Design review of the part built by this model. Coordinates are the model's own, in mm. A direction names the side the tool comes from. Give positions to 0.01 mm unless a question says otherwise; leave off trailing zeros. Loops run counter-clockwise (first coordinate to the right, second up) from the corner with the lowest first, then second, coordinate; pieces in that order, holes last. Notation, with made-up numbers: (-22, -10) -> (-12, -10) arc R28 cw to (-12, 12) -> close; hole circle Ø10 at (3.5, -31). An arc over 180 degrees is marked (long way). Answer in a Markdown table with one row per item. Add a question column.
(1) For line 1 (X direction, y = -7.5, z = 62.5); line 2 (Y direction, x = -4, z = 11); line 3 (X direction, y = -1.5, z = 25.5), list the stretches that pass through material, from the lowest coordinate up.
(2) For pin 1 (6 mm diameter, centred on y = -4.5, z = 82, fed in from +X); pin 2 (5 mm diameter, centred on x = 5.16, z = 92.08, fed in from -Y); pin 3 (4 mm diameter, centred on x = 56.5, z = 35.5, fed in from +Y), all flat-tipped, find the tip position at first contact; note any pin that passes through.
(3) Consider section A-A on y = -4.25. Write out the cut boundary in (x, z).
(4) Draft analysis for pull direction X (two halves, no side actions). For faces 1 (the flat face through (19.5, 0.4, 95.25)), 2 (the cylindrical face through (-0.656, 0.599, 48.292)), 3 (the cylindrical face through (38.095, 0.843, 3.255)), state which applies: +X half, -X half, draft (parallel to the pull), parting line (faces both ways), or undercut.
(5) Consider section C-C on x = 4.5. Write out the cut boundary in (y, z).
(6) Consider section D-D on x = 36.5. Write out the cut boundary in (y, z).
(7) For faces 4 (the cylindrical face through (0.566, -0.597, 48.292)), 5 (the flat face through (55, -11.581, 47)), 6 (the flat face through (-10, -11.581, 47)), list the 3-axis set-ups (+Z, -Z, +X, -X, +Y, -Y) from which the entire face can be reached by the end or side of a thin tool; tool diameter is ignored.
(8) Consider section B-B on z = 42. Write out the cut boundary in (x, y), then the cut area to 3 significant figures.
from build123d import *

# Parameters (mm, degrees)
F1_DEPTH = 95.25
F2_R     = 1.98374
F3_R     = 3.69316
F4_R     = 0.762
F5_R     = 1.8288
F6_DEPTH = 1.70942


with BuildPart() as f1:
    # F0 (on Top) → F1 (new body)
    with BuildSketch(Plane.XY):
        Polygon((0, -13.29058), (0, 0), (45.08116, 0), (45.08116, -13.29058), (61.79058, -13.29058), (61.79058, -11.58116), (46.79058, -11.58116), (46.79058, 1.70942), (-1.70942, 1.70942), (-1.70942, -11.58116), (-16.70942, -11.58116), (-16.70942, -13.29058), align=None)
    extrude(amount=F1_DEPTH)

    # F2
    f2_edges = [f1.edges().sort_by_distance(p)[0] for p in [
        (0, 0, 47.625),
        (-1.70942, -11.58116, 47.625),
        (45.08116, 0, 47.625),
        (46.79058, -11.58116, 47.625),
    ]]
    fillet(f2_edges, radius=F2_R)

    # F3
    f3_edges = [f1.edges().sort_by_distance(p)[0] for p in [
        (0, -13.29058, 47.625),
        (-1.70942, 1.70942, 47.625),
        (46.79058, 1.70942, 47.625),
        (45.08116, -13.29058, 47.625),
    ]]
    fillet(f3_edges, radius=F3_R)

    # F4
    f4_edges = [f1.edges().sort_by_distance(p)[0] for p in [
        (-16.70942, -12.43587, 0),
        (-16.70942, -12.43587, 95.25),
        (61.79058, -12.43587, 0),
        (61.79058, -12.43587, 95.25),
    ]]
    fillet(f4_edges, radius=F4_R)

    # F5 (on face) → F6 (cut, through all)
    with BuildSketch(Plane.XZ):
        with Locations((5.15874, 92.075)):
            Circle(F5_R)
        with Locations((5.15874, 3.175)):
            Circle(F5_R)
        with Locations((39.92242, 92.075)):
            Circle(F5_R)
        with Locations((39.92242, 3.175)):
            Circle(F5_R)
    extrude(amount=-F6_DEPTH, mode=Mode.SUBTRACT)


solid = f1.part
Values follow:
| question | item | result |
|---|---|---|
| 1 | line 1 | -1.71 to 0, 45.08 to 46.79 |
| 1 | line 2 | -13.29 to -11.58 |
| 1 | line 3 | -1.68 to 0.06, 45.02 to 46.76 |
| 2 | pin 1 | x = 46.79 |
| 2 | pin 2 | y = 0 |
| 2 | pin 3 | y = -11.58 |
| 3 | outline | (-1.71, 0) -> (0, 0) -> (0, 95.25) -> (-1.71, 95.25) -> close; (45.08, 0) -> (46.79, 0) -> (46.79, 95.25) -> (45.08, 95.25) -> close |
| 4 | face 1 | draft |
| 4 | face 2 | -X half |
| 4 | face 3 | undercut |
| 5 | outline | (0, 0) -> (1.71, 0) -> (1.71, 1.47) -> (0, 1.47) -> close; (0, 4.88) -> (1.71, 4.88) -> (1.71, 90.37) -> (0, 90.37) -> close; (0, 93.78) -> (1.71, 93.78) -> (1.71, 95.25) -> (0, 95.25) -> close |
| 6 | outline | (0, 0) -> (1.71, 0) -> (1.71, 95.25) -> (0, 95.25) -> close |
| 7 | face 4 | +Z, -Z, -Y |
| 7 | face 5 | +Z, -Z, +X, +Y |
| 7 | face 6 | +Z, -Z, -X, +Y |
| 8 | outline | (-16.71, -13.29) -> (-3.69, -13.29) arc R3.69 ccw to (0, -9.6) -> (0, -1.98) arc R1.98 cw to (1.98, 0) -> (43.1, 0) arc R1.98 cw to (45.08, -1.98) -> (45.08, -9.6) arc R3.69 ccw to (48.77, -13.29) -> (61.79, -13.29) -> (61.79, -11.58) -> (48.77, -11.58) arc R1.98 cw to (46.79, -9.6) -> (46.79, -1.98) arc R3.69 ccw to (43.1, 1.71) -> (1.98, 1.71) arc R3.69 ccw to (-1.71, -1.98) -> (-1.71, -9.6) arc R1.98 cw to (-3.69, -11.58) -> (-16.71, -11.58) -> close |
| 8 | area | 171 mm2 |
